Answer from the drawing. Dimensions are ordinates in mm from the lowest x, y and z of the part. A direction names the side the tool comes from. Give positions to 0.01 mm unless a question says otherwise; leave off trailing zeros. Order: outer loops, then holes, each group sorted by start corner. A loop starts at its lowest first (then second) coordinate and runs counter-clockwise, first axis right, second up. Notation, with made-up numbers: (-39, 8.5) - (-17, 8.5) arc R19 cw to (-17, 19.5) - close; hole circle Ø6 at (46, 8.25). An arc over 180 degrees is marked (long way). Answer in a Markdown table with one row per item. Add a question column.
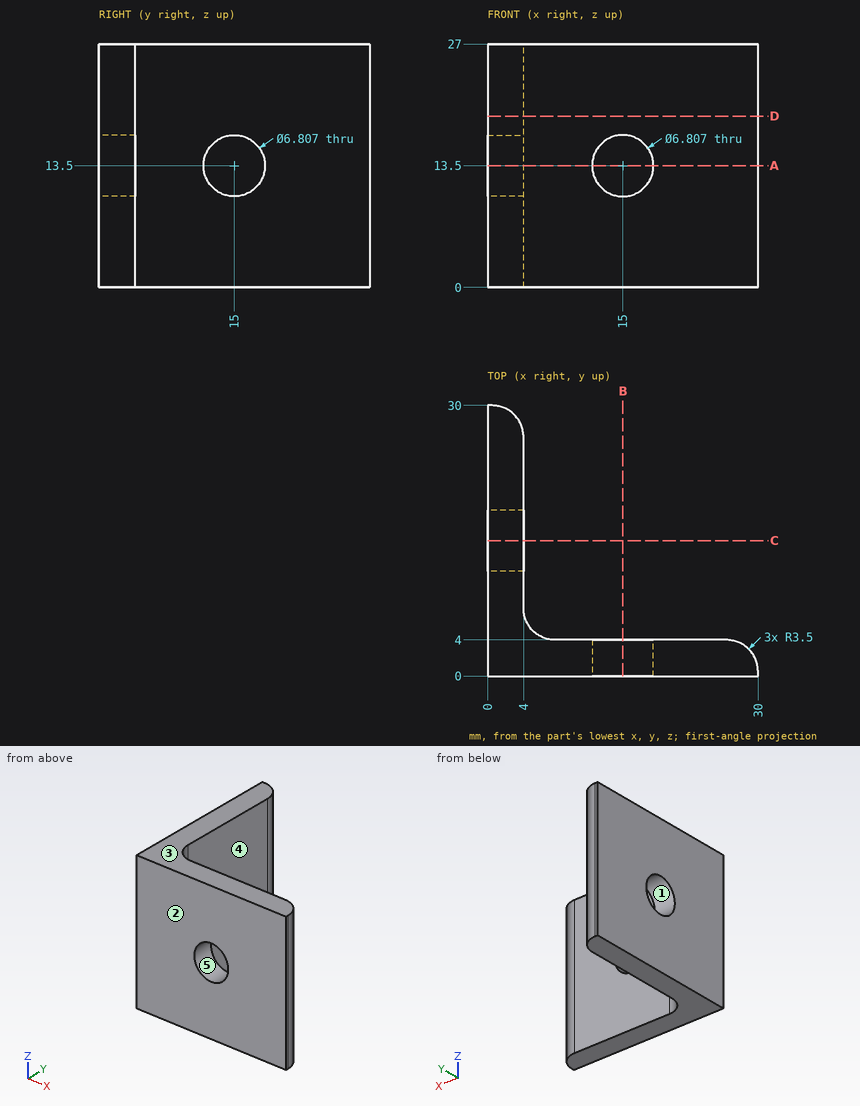
(1) The mould has two halves that part along Z. Classify the marked faces 1, 2 and 3: +Z half, -Z half, draft (parallel to the pull), parting line (faces both ways), or undercut.
(2) For the marked faces 4 and 5, determine the directions among +Z, -Z, +X, -X, +Y, -Y from which every point of the face is accessible in a straight line to the end or side of a thin tool.
(3) Find section D-D, the plane z = 19. Write down the section's boundary in (x, y), plus the area to 3 significant figures.
(4) Straight lines are drawn through the part: line 1 (Z direction, x = 15, y = 2.85); line 2 (Y direction, x = 10.75, z = 3.25). For each, find the intervals that lie inside material, in ascending order.
(5) Each of these flat-tipped pins is pushed along its axis until it touches: P1, Ø1, axis at y = 18, z = 17.5, coming from the +X side; P2, Ø1.5, axis at x = 25.5, z = 7.5, coming from the +Y side. Where does it stop, or does it pass through?
(6) Find section A-A, the plane z = 13.5. Write down the section's boundary in (x, y).
(7) Find section B-B, the plane x = 15. Write down the section's boundary in (y, z).
Answer key:
| question | item | result |
|---|---|---|
| 1 | face 1 | undercut |
| 1 | face 2 | draft |
| 1 | face 3 | +Z half |
| 2 | face 4 | +Z, -Z, +X, +Y |
| 2 | face 5 | +Y, -Y |
| 3 | outline | (0, 0) - (30, 0) - (30, 0.5) arc R3.5 ccw to (26.5, 4) - (7.5, 4) arc R3.5 cw to (4, 7.5) - (4, 26.5) arc R3.5 ccw to (0.5, 30) - (0, 30) - close |
| 3 | area | 221 mm² |
| 4 | line 1 | 0 to 10.1, 16.9 to 27 |
| 4 | line 2 | 0 to 4 |
| 5 | P1 | x = 4 |
| 5 | P2 | y = 4 |
| 6 | outline | (0, 0) - (11.6, 0) - (11.6, 4) - (7.5, 4) arc R3.5 cw to (4, 7.5) - (4, 11.6) - (0, 11.6) - close; (0, 18.4) - (4, 18.4) - (4, 26.5) arc R3.5 ccw to (0.5, 30) - (0, 30) - close; (18.4, 0) - (30, 0) - (30, 0.5) arc R3.5 ccw to (26.5, 4) - (18.4, 4) - close |
| 7 | outline | (0, 0) - (4, 0) - (4, 10.1) - (0, 10.1) - close; (0, 16.9) - (4, 16.9) - (4, 27) - (0, 27) - close |
